For this review, take the finished solid that the model builds, in its own axes (mm). A direction names the side the tool comes from. Give positions to 0.01 mm unless a question says otherwise; leave off trailing zeros. Order: outer loops, then holes, each group sorted by start corner. A loop starts at its lowest first (then second) coordinate and runs counter-clockwise, first axis right, second up. Notation, with made-up numbers: (-17, 24) - (18, 24) arc R19 ccw to (18, 41) - close; hole circle Ø8 at (-10, 48). An arc over 180 degrees is marked (long way). Use a Markdown table: item, result. Add a question column.
1) We need section B-B on x = 15. Write out the cut boundary in (y, z) (3 decimals), then the cut area to 3 significant figures.
2) Clearance check with flat-ended pins moving along their axes: P1, Ø4, axis at x = 18.5, y = 6.5, coming from the -Z side; P2, Ø4, axis at y = 8.5, z = -9.5, coming from the +X side; P3, Ø1, axis at x = 17, y = 12.5, coming from the +Z side. State where each tip first meets the part, or that it passes through.
3) We need section D-D on y = 10.25. Write out the cut boundary in (x, z), then the cut area to 3 significant figures.
4) Mouldability with a two-part tool opening along Y and no side actions: class faces 3 (the face through (1, 0, 7)), 4 (the face through (32.282, 3.348, 3.838)), 5 (the face through (0.128, 8.105, 1.953)) as released by +Y, released by -Y, zero draft, split by the parting line, or undercut.
5) We need section A-A on z = 0. Write out the cut boundary in (x, y) (3 decimals).
6) Wall thickness on L1, parallel to Z at x = 2.5, y = 12.25; L2, parallel to Z at x = 23.5, y = 13; L3, parallel to X at y = 12.5, z = 7: over which ranges is each line inside the solid? List them lowest first.
7) Machinability: for faces 1 (the face through (32, 1.3, 3.8)), 2 (the face through (20, 16, -15)), which of the approach directions +Z, -Z, +X, -X, +Y, -Y give a long, thin tool a straight path to every point of the face, cutting with its end or side? Answer none if there is none.
8) We need section C-C on y = 7. Write out the cut boundary in (x, z) (3 decimals).
```python
from build123d import *


with BuildPart() as part:
    # Çizim1 → Döndür1 (revolve)
    with BuildSketch(Plane.XY, mode=Mode.PRIVATE) as d_nd_r1_sk:
        with BuildLine():
            Line((0, 0.5), (0, 15.5))
            ThreePointArc((0, 15.5), (-0.146446609, 15.853553391), (-0.5, 16))
            Line((-0.5, 16), (-6.975, 16))
            ThreePointArc((-6.975, 16), (-7.365434405, 15.812347524), (-7.462804878, 15.390243902))
            Line((-7.462804878, 15.390243902), (-7.033242887, 13.481079498))
            Line((-7.033242887, 13.481079498), (-5.082023375, 13.920103888))
            Line((-5.082023375, 13.920103888), (-2.251352946, 1.339346427))
            Line((-2.251352946, 1.339346427), (-4.202572458, 0.900322037))
            Line((-4.202572458, 0.900322037), (-4.087804878, 0.390243902))
            ThreePointArc((-4.087804878, 0.390243902), (-3.912347524, 0.109565595), (-3.6, 0))
            Line((-3.6, 0), (-0.5, 0))
            ThreePointArc((-0.5, 0), (-0.146446609, 0.146446609), (0, 0.5))
        make_face()
    revolve(d_nd_r1_sk.sketch.rotate(Axis((15, 1.339346427, 0), (0, 1, 0)), 270), axis=Axis((15, 1.339346427, 0), (0, 1, 0)))


solid = part.part
```
Checked values:
| question | item | result |
|---|---|---|
| 1 | outline | (0, -18.6) arc R0.5 ccw to (0.39, -19.088) - (0.9, -19.203) - (1.339, -17.251) - (13.92, -20.082) - (13.481, -22.033) - (15.39, -22.463) arc R0.5 ccw to (16, -21.975) - (16, -15.5) arc R0.5 ccw to (15.5, -15) - (0.5, -15) arc R0.5 ccw to (0, -15.5) - close; (0, 15.5) arc R0.5 ccw to (0.5, 15) - (15.5, 15) arc R0.5 ccw to (16, 15.5) - (16, 21.975) arc R0.5 ccw to (15.39, 22.463) - (13.481, 22.033) - (13.92, 20.082) - (1.339, 17.251) - (0.9, 19.203) - (0.39, 19.088) arc R0.5 ccw to (0, 18.6) - close |
| 1 | area | 134 mm² |
| 2 | P1 | z = -18.64 |
| 2 | P2 | x = 32.44 |
| 2 | P3 | z = 19.78 |
| 3 | outline | circle Ø38.51 at (15, 0); hole circle Ø30 at (15, 0) |
| 3 | area | 458 mm² |
| 4 | face 3 | released by -Y |
| 4 | face 4 | undercut |
| 4 | face 5 | zero draft |
| 5 | outline | (-7.463, 15.39) - (-7.033, 13.481) - (-5.082, 13.92) - (-2.251, 1.339) - (-4.203, 0.9) - (-4.088, 0.39) arc R0.5 ccw to (-3.6, 0) - (-0.5, 0) arc R0.5 ccw to (0, 0.5) - (0, 15.5) arc R0.5 ccw to (-0.5, 16) - (-6.975, 16) arc R0.5 ccw to start; (30, 0.5) arc R0.5 ccw to (30.5, 0) - (33.6, 0) arc R0.5 ccw to (34.088, 0.39) - (34.203, 0.9) - (32.251, 1.339) - (35.082, 13.92) - (37.033, 13.481) - (37.463, 15.39) arc R0.5 ccw to (36.975, 16) - (30.5, 16) arc R0.5 ccw to (30, 15.5) - close |
| 6 | L1 | -15.23 to -8.29, 8.29 to 15.23 |
| 6 | L2 | -17.97 to -12.36, 12.36 to 17.97 |
| 6 | L3 | -3.48 to 1.73, 28.27 to 33.48 |
| 7 | face 1 | none |
| 7 | face 2 | +Z, -Z, +X, -X, +Y |
| 8 | outline | circle Ø37.05 at (15, 0); hole circle Ø30 at (15, 0) |
